Read the model definition and answer for the solid it produces. Units are mm, in the model's axes. A direction names the side the tool comes from. Coordinates: 2 decimals unless noted, no trailing zeros. Write each loop counter-clockwise with the first axis right and the second up, starting at its lowest first coordinate (ties: lowest second). Pieces come first, ordered by that corner, then holes. Notation, with made-up numbers: (-30, 86.25) -> (2, 86.25) arc R23 ccw to (2, 99.25) -> close; hole circle Ø3 at (58.5, 56). An arc over 180 degrees is marked (long way). One line per item, written item: value. Start each with the question number.
1. Find section A-A, the plane y = 4.5. State how many separate pieces and enclosed holes the cut face has, and give its area (3 significant figures).
2. Given P1, Ø5, axis at x = 17, y = 4, coming from the +Z side; P2, Ø2, axis at x = 11.5, y = 2.5, coming from the -Z side, each flat-ended and moving along its own axis, determine where each tip first touches the part or whether it passes through.
3. Find section D-D, the plane z = -11.5. Write down the section's boundary in (x, y), and give its area (3 significant figures).
4. For faces 1 (the flat face through (3.969, 6, -10)), 2 (the flat face through (0, 6, -6)), determine the directions among +Z, -Z, +X, -X, +Y, -Y from which every point of the face is accessible in a straight line to the end or side of a thin tool.
5. For a pull along Z with two mould halves and no side action, classify faces 3 (the cylindrical face through (1.66, 6.44, -5.15)), 4 (the flat face through (2, 6, -12.7)), 5 (the flat face through (9, 12.7, -6)) as pulls with the +Z half, pulls with the -Z half, needs draft (parallel to the pull), parting line crosses it, or undercut.
6. Consider line 1 along X through (y, z) = (1, -3.25); line 2 along X through (y, z) = (3, -8.75); line 3 along X through (y, z) = (2.25, -1). Determine where each line is inside the solid, lowest interval first.
7. Find section C-C, the plane x = 12. Write down the section's boundary in (y, z).
8. Find section B-B, the plane z = -1.75. Write down the section's boundary in (x, y) (3 decimals), and give its area (3 significant figures).
```python
from build123d import *

# Parameters (mm, degrees)
SKETCH1_W           = 19.05
SKETCH1_H           = 12.7
BOSS_EXTRUDE1_DEPTH = 12.7
SKETCH2_R           = 2.4892
SKETCH2_W           = 11.1125
SKETCH2_H           = 4.7625
CUT_EXTRUDE1_DEPTH  = 12.7
SKETCH3_R           = 3.2639
CUT_EXTRUDE2_DEPTH  = 12.7


with BuildPart() as part:
    # Sketch1 → Boss-Extrude1 (new body)
    with BuildSketch(Plane(origin=(0, 0, 0), x_dir=(1, 0, 0), z_dir=(0, 1, 0))):
        with Locations((9.525, 6.35)):
            Rectangle(SKETCH1_W, SKETCH1_H)
    extrude(amount=BOSS_EXTRUDE1_DEPTH)

    # Sketch2 → Cut-Extrude1 (cut)
    with BuildSketch(Plane(origin=(0, 12.7, 0), x_dir=(1, 0, 0), z_dir=(0, 1, 0))):
        with Locations(Location((3.175, 3.175, 0), (0, 0, 270))):
            Circle(SKETCH2_R)
        with Locations(Location((15.875, 3.175, 0), (0, 0, 270))):
            Circle(SKETCH2_R)
        with Locations((9.525, 10.31875)):
            Rectangle(SKETCH2_W, SKETCH2_H)
    extrude(amount=-CUT_EXTRUDE1_DEPTH, mode=Mode.SUBTRACT)

    # Sketch3 → Cut-Extrude2 (cut)
    with BuildSketch(Plane.XY):
        with Locations((9.525, 6.35)):
            Circle(SKETCH3_R)
    extrude(amount=-CUT_EXTRUDE2_DEPTH, mode=Mode.SUBTRACT)


solid = part.part
```
Answer block:
1. separate pieces: 2
1. enclosed holes: 2
1. area: 107 mm2
2. P1: stops at z = 0
2. P2: stops at z = -7.94
3. outline: (0, 0) -> (3.97, 0) -> (3.97, 12.7) -> (0, 12.7) -> close; (15.08, 0) -> (19.05, 0) -> (19.05, 12.7) -> (15.08, 12.7) -> close
3. area: 101 mm2
4. face 1: -Z, +Y, -Y
4. face 2: +Z, -Z, -X, +Y, -Y
5. face 3: undercut
5. face 4: pulls with the -Z half
5. face 5: needs draft
6. line 1: x = 0 to 0.69, 5.66 to 13.39, 18.36 to 19.05
6. line 2: x = 0 to 3.97, 15.08 to 19.05
6. line 3: x = 0 to 1.96, 4.39 to 14.66, 17.09 to 19.05
7. outline: (0, -7.94) -> (4.22, -7.94) -> (4.22, 0) -> (0, 0) -> close; (8.48, -7.94) -> (12.7, -7.94) -> (12.7, 0) -> (8.48, 0) -> close
8. outline: (0, 0) -> (1.134, 0) -> (1.134, 12.7) -> (0, 12.7) -> close; (5.216, 0) -> (13.834, 0) -> (13.834, 12.7) -> (5.216, 12.7) -> close; (17.916, 0) -> (19.05, 0) -> (19.05, 12.7) -> (17.916, 12.7) -> close; hole circle Ø6.528 at (9.525, 6.35)
8. area: 105 mm2
